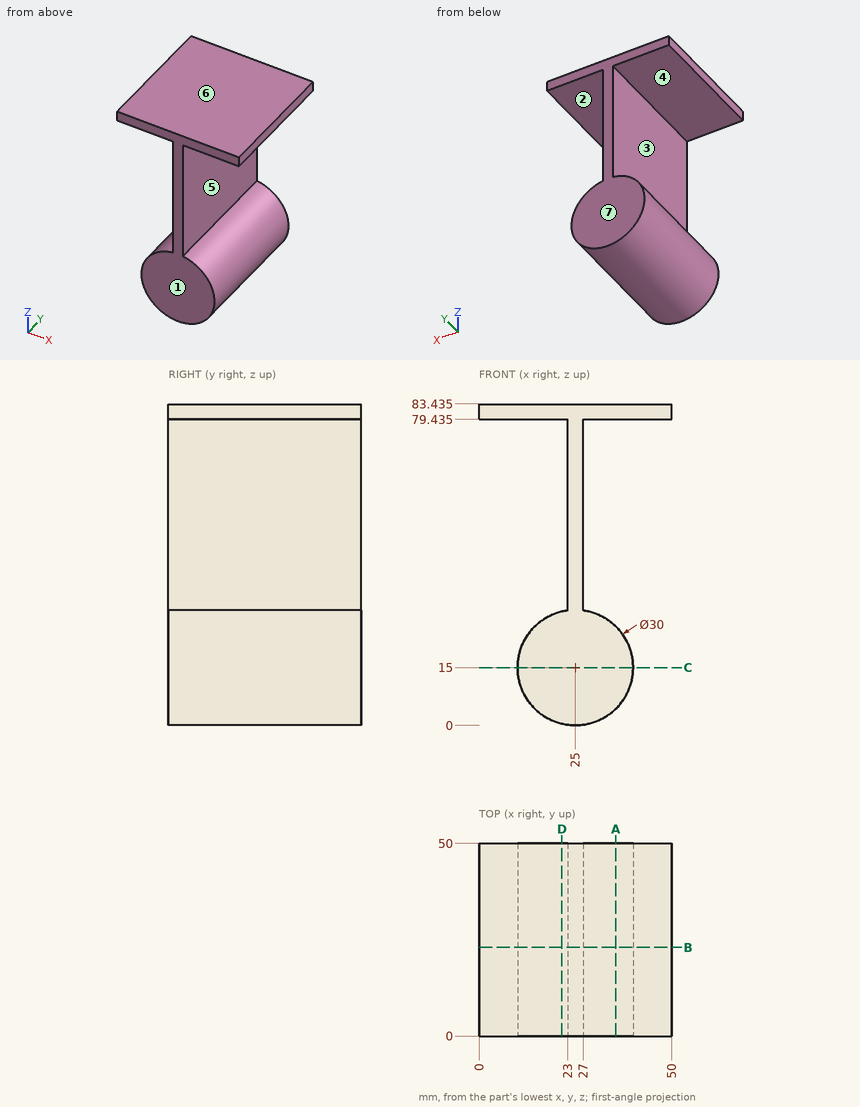
The figure shows three views and two pictorial views of one solid part (mm, origin at its lowest corner). Answer the questions. A direction names the side the tool comes from. Give positions to 0.01 mm unless a question says otherwise; leave off trailing zeros. Write each loop counter-clockwise with the first axis right and the second up, starting at its lowest first coordinate (ties: lowest second). Pieces come first, ordered by that corner, then holes. Notation, with made-up numbers: (68, 5.5) - (97, 5.5) arc R17 cw to (97, 20.5) - close; hole circle Ø11 at (20, -16). An arc over 180 degrees is marked (long way). Use one line per item in the form item = value. Start each with the question number.
1) A tool of negligible diameter and unlimited length cuts with its end or side. For the marked faces 1, 2 and 3, from which of +Z, -Z, +X, -X, +Y, -Y can it reach the whole face along a straight path? Write none if from no direction.
2) Flat-ended cylindrical pins translate along their axes: pin 1 Ø1.5 at (y, z) = (10.5, 74) entering from -X; pin 2 Ø1.5 at (y, z) = (31.5, 31) entering from +X; pin 3 Ø18.5 at (x, y) = (9.5, 32) entering from -Z (1 decimal). Find the tip coordinate at first contact, or state that the pin passes through.
3) Consider line 1 along X through (y, z) = (25.5, 31); line 2 along Z through (x, y) = (3, 5.5) (1 decimal); line 3 along Z through (x, y) = (29, 5) (1 decimal). Determine where each line is inside the solid, lowest interval first. Write a range as from..to.
4) Find section B-B on y = 23. Determine the outline of the cut face in (x, z) (1 decimal), plus the area to 4 significant figures.
5) Find section A-A on x = 35.5. Determine the outline of the cut face in (y, z) (1 decimal).
6) Find section D-D on x = 21.5. Determine the outline of the cut face in (y, z) (1 decimal), plus the area to 3 significant figures.
7) The mould has two halves that part along Z. Classify the marked faces 4, 5, 6 and 7: pulls with the +Z half, pulls with the -Z half, needs draft (parallel to the pull), parting line crosses it, or undercut.
8) Find section C-C on z = 15. Determine the outline of the cut face in (x, y).
Geometry results:
q1.face_1 = +Z, -Z, +X, -X, -Y
q1.face_2 = +X, +Y, -Y
q1.face_3 = -X, +Y, -Y
q2.pin_1 = 23
q2.pin_2 = 27
q2.pin_3 = 1.4
q3.line_1 = 23..27
q3.line_2 = 79.4..83.4
q3.line_3 = 0.5..29.5, 79.4..83.4
q4.outline = (0, 79.4) - (23, 79.4) - (23, 29.9) arc R15 ccw (long way) to (27, 29.9) - (27, 79.4) - (50, 79.4) - (50, 83.4) - (0, 83.4) - close
q4.area = 1,105 mm2
q5.outline = (0, 4.3) - (50, 4.3) - (50, 25.7) - (0, 25.7) - close; (0, 79.4) - (50, 79.4) - (50, 83.4) - (0, 83.4) - close
q6.outline = (0, 0.4) - (50, 0.4) - (50, 29.6) - (0, 29.6) - close; (0, 79.4) - (50, 79.4) - (50, 83.4) - (0, 83.4) - close
q6.area = 1,660 mm2
q7.face_4 = undercut
q7.face_5 = undercut
q7.face_6 = pulls with the +Z half
q7.face_7 = needs draft
q8.outline = (10, 0) - (40, 0) - (40, 50) - (10, 50) - close
